Verification items for the finished model (mm, model axes). Round coordinates to 2 decimals unless told otherwise and drop trailing zeros. Write each loop counter-clockwise with the first axis right and the second up, starting at its lowest first coordinate (ties: lowest second). Pieces come first, ordered by that corner, then holes. Notation, with made-up numbers: M -13.5,89.25 L 43.5,89.25 A26 ccw 43.5,124.25 Z; hole C 3.25,83.5 d9. An arc over 180 degrees is marked long. One line per item, written item: value. Start each with the question number.
Item 1: Gauge pin test, flat ends, axial feed: pin 1 (1.5 mm diameter, centred on y = 78, z = -5, fed in from -X); pin 2 (3 mm diameter, centred on y = 111, z = -2, fed in from +X); pin 3 (5 mm diameter, centred on x = 5, y = 86, fed in from -Z). Record the tip position at first contact, or that the pin passes through.
Item 2: Draft check along Z on faces 1 (the face through (6.466, 73.028, 2.681)), 2 (the face through (4, 0, 6)), 3 (the face through (-1.73, 73.03, 7.81)). Enter one of: +Z half, -Z half, draft (parallel to the pull), parting line (faces both ways), or undercut.
Item 3: Section check C-C, the plane y = 103.5. Record the cut outline in (x, z).
Item 4: Thickness scan on probe 1 along Y at (x, z) = (0, 7.5); probe 2 along X at (y, z) = (105.5, 0); probe 3 along Z at (x, y) = (-3.5, 92.5). Record the ranges inside material, lowest first. Write a range as from..to.
Item 5: Section check A-A, the plane z = 0. Record the cut outline in (x, y).
Item 6: Section check B-B, the plane x = 2. Record the cut outline in (y, z), then the cut area to 3 significant figures.
from build123d import *

# Parameters (mm, degrees)
SKETCH2_R           = 8
SKETCH2_R_2         = 7
BOSS_EXTRUDE1_DEPTH = 148.12915224
M2_TAPPED_HOLE1_D   = 1.6


with BuildPart() as part:
    # Sketch2 → Boss-Extrude1 (new body)
    with BuildSketch(Plane(origin=(0, 0, 0), x_dir=(1, 0, 0), z_dir=(0, 1, 0))):
        Circle(SKETCH2_R)
        Circle(SKETCH2_R_2, mode=Mode.SUBTRACT)
    extrude(amount=BOSS_EXTRUDE1_DEPTH)

    # M2 Tapped Hole1 (through all)
    with Locations(Plane.XY.offset(8)):
        with Locations((0, 11), (0, 138.27915224)):
            Hole(M2_TAPPED_HOLE1_D / 2)


solid = part.part
Response values:
1. pin 1: stops at x = -6.78
1. pin 2: stops at x = 7.98
1. pin 3: stops at z = -7.6
2. face 1: undercut
2. face 2: draft
2. face 3: parting line
3. outline: C 0,0 d16; hole C 0,0 d14
4. probe 1: y = 0..10.2, 11.8..137.48, 139.08..148.13
4. probe 2: x = -8..-7, 7..8
4. probe 3: z = -7.19..-6.06, 6.06..7.19
5. outline: M -8,0 L -7,0 L -7,148.13 L -8,148.13 Z; M 7,0 L 8,0 L 8,148.13 L 7,148.13 Z
6. outline: M 0,-7.75 L 148.13,-7.75 L 148.13,-6.71 L 0,-6.71 Z; M 0,6.71 L 148.13,6.71 L 148.13,7.75 L 0,7.75 Z
6. area: 307 mm2
